Part model, mm, in its own coordinate system. Coordinates: 2 decimals unless noted, no trailing zeros. Order: outer loops, then holes, each group sorted by start corner. A loop starts at its lowest first (then second) coordinate and runs counter-clockwise, first axis right, second up.
from build123d import *

# Parameters (mm, degrees)
SKETCH1_W                    = 3.175
SKETCH1_H                    = 12.7
MAIN_EXTRUDE_DEPTH           = 3.175
SKETCH8_R                    = 1.5
SKETCH8_W                    = 3.175
SKETCH8_H                    = 31.877
MOUNT_HOLES_DEPTH            = 4.175
DOOR_SLOTS_DEPTH             = 4.175
SKETCH4_W                    = 30.099999998
SKETCH4_H                    = 16.699
TROUGH_AND_LEVER_HOLES_DEPTH = 4.175
SKETCH10_R                   = 1.5
DOOR_GUIDE_MOUNT_HOLES_DEPTH = 4.175
SKETCH12_R                   = 1.5
EXTENSION_CLIP_HOLES_DEPTH   = 4.175
EXTENSION_CENTER_CUT_DEPTH   = 4.175


with BuildPart() as part:
    # Sketch1 → Main Extrude (new body)
    with BuildSketch(Plane.XY):
        Polygon((-243.84, -134.112), (-189.653333333, -134.112), (-189.653333333, -139.7), (-135.466666667, -139.7), (-135.466666667, -134.112), (-81.28, -134.112), (-81.28, -139.7), (-27.093333333, -139.7), (-27.093333333, -134.112), (27.093333333, -134.112), (27.093333333, -139.7), (81.28, -139.7), (81.28, -134.112), (135.466666667, -134.112), (135.466666667, -139.7), (189.653333333, -139.7), (189.653333333, -134.112), (243.84, -134.112), (243.84, -139.7), (298.026666667, -139.7), (298.026666667, -134.112), (352.213333333, -134.112), (352.213333333, -139.7), (406.4, -139.7), (406.4, 139.7), (381, 139.7), (381, 127), (377.825, 127), (377.825, 139.7), (-377.825, 139.7), (-377.825, 127), (-381, 127), (-381, 139.7), (-406.4, 139.7), (-406.4, -139.7), (-352.213333333, -139.7), (-352.213333333, -134.112), (-298.026666667, -134.112), (-298.026666667, -139.7), (-243.84, -139.7), align=None)
        with Locations((-379.4125, -120.65)):
            Rectangle(SKETCH1_W, SKETCH1_H, mode=Mode.SUBTRACT)
        with Locations((-379.4125, -95.25)):
            Rectangle(SKETCH1_W, SKETCH1_H, mode=Mode.SUBTRACT)
        with Locations((379.4125, 82.55)):
            Rectangle(SKETCH1_W, SKETCH1_H, mode=Mode.SUBTRACT)
        with Locations((379.4125, 57.15)):
            Rectangle(SKETCH1_W, SKETCH1_H, mode=Mode.SUBTRACT)
        with Locations((379.4125, 31.75)):
            Rectangle(SKETCH1_W, SKETCH1_H, mode=Mode.SUBTRACT)
        with Locations((379.4125, 6.35)):
            Rectangle(SKETCH1_W, SKETCH1_H, mode=Mode.SUBTRACT)
        with Locations((379.4125, -19.05)):
            Rectangle(SKETCH1_W, SKETCH1_H, mode=Mode.SUBTRACT)
        with Locations((379.4125, -44.45)):
            Rectangle(SKETCH1_W, SKETCH1_H, mode=Mode.SUBTRACT)
        with Locations((379.4125, -69.85)):
            Rectangle(SKETCH1_W, SKETCH1_H, mode=Mode.SUBTRACT)
        with Locations((379.4125, -95.25)):
            Rectangle(SKETCH1_W, SKETCH1_H, mode=Mode.SUBTRACT)
        with Locations((379.4125, -120.65)):
            Rectangle(SKETCH1_W, SKETCH1_H, mode=Mode.SUBTRACT)
        with Locations((-379.4125, -69.85)):
            Rectangle(SKETCH1_W, SKETCH1_H, mode=Mode.SUBTRACT)
        with Locations((-379.4125, -44.45)):
            Rectangle(SKETCH1_W, SKETCH1_H, mode=Mode.SUBTRACT)
        with Locations((-379.4125, -19.05)):
            Rectangle(SKETCH1_W, SKETCH1_H, mode=Mode.SUBTRACT)
        with Locations((-379.4125, 6.35)):
            Rectangle(SKETCH1_W, SKETCH1_H, mode=Mode.SUBTRACT)
        with Locations((-379.4125, 31.75)):
            Rectangle(SKETCH1_W, SKETCH1_H, mode=Mode.SUBTRACT)
        with Locations((-379.4125, 57.15)):
            Rectangle(SKETCH1_W, SKETCH1_H, mode=Mode.SUBTRACT)
        with Locations((-379.4125, 82.55)):
            Rectangle(SKETCH1_W, SKETCH1_H, mode=Mode.SUBTRACT)
        with Locations((-379.4125, 107.95)):
            Rectangle(SKETCH1_W, SKETCH1_H, mode=Mode.SUBTRACT)
        with Locations((379.4125, 107.95)):
            Rectangle(SKETCH1_W, SKETCH1_H, mode=Mode.SUBTRACT)
    extrude(amount=MAIN_EXTRUDE_DEPTH)

    # Sketch8 → Mount Holes (cut, through all)
    with BuildSketch(Plane.XY.offset(3.175)):
        with Locations((-393.7, -120.65)):
            Circle(SKETCH8_R)
        with Locations((393.7, -120.65)):
            Circle(SKETCH8_R)
        with Locations((-382.5875, 12.319)):
            Rectangle(SKETCH8_W, SKETCH8_H)
        with Locations((382.5875, 12.319)):
            Rectangle(SKETCH8_W, SKETCH8_H)
    extrude(amount=-MOUNT_HOLES_DEPTH, mode=Mode.SUBTRACT)

    # Sketch3 → Door Slots (cut, through all)
    with BuildSketch(Plane.XY.offset(3.175)):
        Polygon((-88.7095, 126.492), (-92.6465, 126.492), (-92.6465, 82.042), (-96.52, 82.042), (-96.52, 10.3505), (-106.553, 10.3505), (-106.553, 0.8255), (-96.52, 0.8255), (-96.52, -134.112), (-84.836, -134.112), (-84.836, 0.8255), (-74.803, 0.8255), (-74.803, 10.3505), (-84.836, 10.3505), (-84.836, 82.042), (-88.7095, 82.042), align=None)
        Polygon((92.6465, 126.492), (88.7095, 126.492), (88.7095, 82.042), (84.836, 82.042), (84.836, 10.3505), (74.803, 10.3505), (74.803, 0.8255), (84.836, 0.8255), (84.836, -134.112), (96.52, -134.112), (96.52, 0.8255), (106.553, 0.8255), (106.553, 10.3505), (96.52, 10.3505), (96.52, 82.042), (92.6465, 82.042), align=None)
    extrude(amount=-DOOR_SLOTS_DEPTH, mode=Mode.SUBTRACT)

    # Sketch4 → Trough and Lever Holes (cut, through all)
    with BuildSketch(Plane.XY):
        Polygon((-52.178, -134.112), (-52.178, -139.7), (-2.178, -139.7), (-2.178, -134.112), (1.124, -134.112), (1.124, -112.40999997), (-2.178, -112.40999997), (-2.178, -101.792), (-52.178, -101.792), (-52.178, -112.40999997), (-55.48, -112.40999997), (-55.48, -134.112), align=None)
        with Locations((27.178, -110.1415)):
            Rectangle(SKETCH4_W, SKETCH4_H)
    extrude(amount=TROUGH_AND_LEVER_HOLES_DEPTH, mode=Mode.SUBTRACT)

    # Sketch10 → Door Guide Mount Holes (cut, through all)
    with BuildSketch(Plane.XY.offset(3.175)):
        with Locations((-101.678, 127.492)):
            Circle(SKETCH10_R)
        with Locations((-79.678, 127.492)):
            Circle(SKETCH10_R)
        with Locations((79.678, 127.492)):
            Circle(SKETCH10_R)
        with Locations((101.678, 127.492)):
            Circle(SKETCH10_R)
    extrude(amount=-DOOR_GUIDE_MOUNT_HOLES_DEPTH, mode=Mode.SUBTRACT)

    # Sketch12 → Extension Clip Holes (cut, through all)
    with BuildSketch(Plane.XY.offset(3.175)):
        with Locations((-246.507, 20.193)):
            Circle(SKETCH12_R)
        with Locations((-246.507, 4.445)):
            Circle(SKETCH12_R)
        with Locations((-221.107, 4.445)):
            Circle(SKETCH12_R)
        with Locations((-221.107, 20.193)):
            Circle(SKETCH12_R)
        with Locations((-243.332, 133.35)):
            Circle(SKETCH12_R)
        with Locations((-224.282, 133.35)):
            Circle(SKETCH12_R)
        with Locations((224.282, 133.35)):
            Circle(SKETCH12_R)
        with Locations((243.332, 133.35)):
            Circle(SKETCH12_R)
        with Locations((221.107, 20.193)):
            Circle(SKETCH12_R)
        with Locations((221.107, 4.445)):
            Circle(SKETCH12_R)
        with Locations((246.507, 4.445)):
            Circle(SKETCH12_R)
        with Locations((246.507, 20.193)):
            Circle(SKETCH12_R)
    extrude(amount=-EXTENSION_CLIP_HOLES_DEPTH, mode=Mode.SUBTRACT)

    # Sketch11_3 → Extension Center Cut (cut, through all)
    with BuildSketch(Plane.XY.offset(3.175)):
        Polygon((-232.2195, 127), (-232.2195, 139.7), (-406.4, 139.7), (-406.4, -139.7), (-235.3945, -139.7), (-235.3945, -127), (-232.2195, -127), (-232.2195, -114.3), (-235.3945, -114.3), (-235.3945, -101.6), (-232.2195, -101.6), (-232.2195, -88.9), (-235.3945, -88.9), (-235.3945, -76.2), (-232.2195, -76.2), (-232.2195, -63.5), (-235.3945, -63.5), (-235.3945, -50.8), (-232.2195, -50.8), (-232.2195, -38.1), (-235.3945, -38.1), (-235.3945, -25.4), (-232.2195, -25.4), (-232.2195, -12.7), (-235.3945, -12.7), (-235.3945, 0), (-232.2195, 0), (-232.2195, 12.7), (-235.3945, 12.7), (-235.3945, 25.4), (-232.2195, 25.4), (-232.2195, 38.1), (-235.3945, 38.1), (-235.3945, 50.8), (-232.2195, 50.8), (-232.2195, 63.5), (-235.3945, 63.5), (-235.3945, 76.2), (-232.2195, 76.2), (-232.2195, 88.9), (-235.3945, 88.9), (-235.3945, 101.6), (-232.2195, 101.6), (-232.2195, 114.3), (-235.3945, 114.3), (-235.3945, 127), align=None)
        Polygon((406.4, 139.7), (232.2195, 139.7), (232.2195, 127), (235.3945, 127), (235.3945, 114.3), (232.2195, 114.3), (232.2195, 101.6), (235.3945, 101.6), (235.3945, 88.9), (232.2195, 88.9), (232.2195, 76.2), (235.3945, 76.2), (235.3945, 63.5), (232.2195, 63.5), (232.2195, 50.8), (235.3945, 50.8), (235.3945, 38.1), (232.2195, 38.1), (232.2195, 25.4), (235.3945, 25.4), (235.3945, 12.7), (232.2195, 12.7), (232.2195, 0), (235.3945, 0), (235.3945, -12.7), (232.2195, -12.7), (232.2195, -25.4), (235.3945, -25.4), (235.3945, -38.1), (232.2195, -38.1), (232.2195, -50.8), (235.3945, -50.8), (235.3945, -63.5), (232.2195, -63.5), (232.2195, -76.2), (235.3945, -76.2), (235.3945, -88.9), (232.2195, -88.9), (232.2195, -101.6), (235.3945, -101.6), (235.3945, -114.3), (232.2195, -114.3), (232.2195, -127), (235.3945, -127), (235.3945, -139.7), (406.4, -139.7), align=None)
    extrude(amount=-EXTENSION_CENTER_CUT_DEPTH, mode=Mode.SUBTRACT)


solid = part.part
Q1. Pin check, flat tips, straight feed: pin 1 Ø1 at (x, z) = (-233, 1.5) entering from +Y; pin 2 Ø1 at (y, z) = (32, 1) entering from +X; pin 3 Ø1.6 at (y, z) = (-137, 1.5) entering from +X. Stop position of each tip, or through.
Results list:
pin 1: stops at y = 127
pin 2: stops at x = 232.22
pin 3: stops at x = 189.65
Q2. Cut at C-C on x = -115.5. Write the cut outline in (y, z) (3 decimals).
Results list:
outline: (-134.112, 0) - (139.7, 0) - (139.7, 3.175) - (-134.112, 3.175) - close
Q3. Cut at D-D on z = 2.1. Count the separate pieces of the cut face and the enclosed holes in it, and give its area (3 significant figures).
Results list:
separate pieces: 1
enclosed holes: 11
area: 121,000 mm2
Q4. Cut at A-A on y = -95. Write the cut outline in (x, z) (1 decimal).
Results list:
outline: (-232.2, 0) - (-96.5, 0) - (-96.5, 3.2) - (-232.2, 3.2) - close; (-84.8, 0) - (84.8, 0) - (84.8, 3.2) - (-84.8, 3.2) - close; (96.5, 0) - (232.2, 0) - (232.2, 3.2) - (96.5, 3.2) - close
Q5. Cut at B-B on y = 71. Write the cut outline in (x, z) (1 decimal).
Results list:
outline: (-235.4, 0) - (-96.5, 0) - (-96.5, 3.2) - (-235.4, 3.2) - close; (-84.8, 0) - (84.8, 0) - (84.8, 3.2) - (-84.8, 3.2) - close; (96.5, 0) - (235.4, 0) - (235.4, 3.2) - (96.5, 3.2) - close
Q6. Wall check: line 1 along X through (y, z) = (-20.5, 2.95); line 2 along X through (y, z) = (107, 2.65); line 3 along Y through (x, z) = (13.5, 0.7). Give the ranges that are in metal, low to high.
Results list:
line 1: x = -232.22 to -96.52, -84.84 to 84.84, 96.52 to 232.22
line 2: x = -232.22 to -92.65, -88.71 to 88.71, 92.65 to 232.22
line 3: y = -134.11 to -118.49, -101.79 to 139.7
